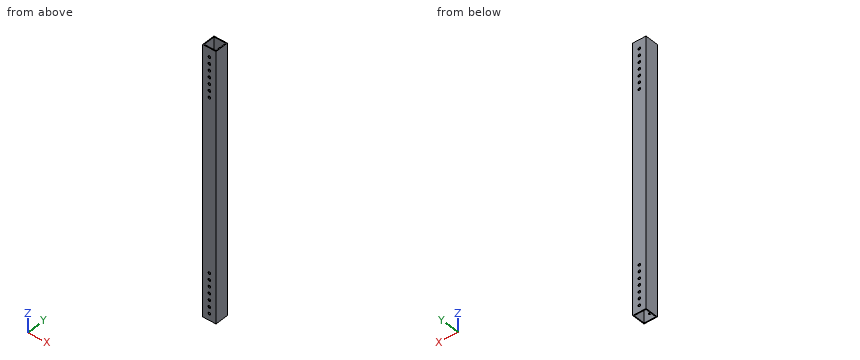
from build123d import *

# Parameters (mm, degrees)
SKETCH1_W               = 25.4
SKETCH1_H               = 25.4
BOSS_EXTRUDE1_DEPTH     = 256.145698528
SHELL1_T                = -1.5875
CUT_EXTRUDE1_DEPTH      = 257.774607145
CUT_EXTRUDE1_DEPTH_BACK = 257.774607145
SKETCH3_R               = 2.4892


with BuildPart() as part:
    # Sketch1 → Boss-Extrude1 (new, symmetric)
    with BuildSketch(Plane.XY):
        Rectangle(SKETCH1_W, SKETCH1_H)
    extrude(amount=BOSS_EXTRUDE1_DEPTH, both=True)

    # Shell1
    shell1_openings = [part.faces().sort_by_distance(p)[0] for p in [
        (0, 0, 256.145698528),
        (0, 0, -256.145698528),
    ]]
    offset(amount=SHELL1_T, openings=shell1_openings, kind=Kind.INTERSECTION)

    # Sketch3 → Cut-Extrude1 (cut, two sides: drawn at the far end of the back side and taken through both)
    with BuildSketch(Plane(origin=(0, 0, 0), x_dir=(1, 0, 0), z_dir=(0, 1, 0)).offset(-CUT_EXTRUDE1_DEPTH_BACK)):
        with Locations(Location((0, 243.445698528, 0), (0, 0, 270))):
            Circle(SKETCH3_R)
        with Locations(Location((0, 230.745698528, 0), (0, 0, 270))):
            Circle(SKETCH3_R)
        with Locations(Location((0, 218.045698528, 0), (0, 0, 270))):
            Circle(SKETCH3_R)
        with Locations(Location((0, 205.345698528, 0), (0, 0, 270))):
            Circle(SKETCH3_R)
        with Locations(Location((0, 192.645698528, 0), (0, 0, 270))):
            Circle(SKETCH3_R)
        with Locations(Location((0, 179.945698528, 0), (0, 0, 270))):
            Circle(SKETCH3_R)
        with Locations(Location((0, 167.245698528, 0), (0, 0, 270))):
            Circle(SKETCH3_R)
        with Locations(Location((0, -162.954301472, 0), (0, 0, 270))):
            Circle(SKETCH3_R)
        with Locations(Location((0, -175.654301472, 0), (0, 0, 270))):
            Circle(SKETCH3_R)
        with Locations(Location((0, -188.354301472, 0), (0, 0, 270))):
            Circle(SKETCH3_R)
        with Locations(Location((0, -201.054301472, 0), (0, 0, 270))):
            Circle(SKETCH3_R)
        with Locations(Location((0, -213.754301472, 0), (0, 0, 270))):
            Circle(SKETCH3_R)
        with Locations(Location((0, -226.454301472, 0), (0, 0, 270))):
            Circle(SKETCH3_R)
        with Locations(Location((0, -239.154301472, 0), (0, 0, 270))):
            Circle(SKETCH3_R)
    extrude(amount=CUT_EXTRUDE1_DEPTH + CUT_EXTRUDE1_DEPTH_BACK, mode=Mode.SUBTRACT)


solid = part.part
Geometry: final body of the model. Coordinates: model frame, mm. Round coordinates to 2 decimals unless told otherwise and drop trailing zeros. Order: outer loops, then holes, each group sorted by start corner. A loop starts at its lowest first (then second) coordinate and runs counter-clockwise, first axis right, second up.
Q1. Material intervals for probe 1 along X at (y, z) = (1, -166.5), sorted ascending.
Result sheet:
probe 1: x = -12.7 to -11.11, 11.11 to 12.7
Q2. Section A-A, the plane x = -6.75. Output: boundary loops of the cut face in (y, z).
Result sheet:
outline: (-12.7, -256.15) - (-11.11, -256.15) - (-11.11, 256.15) - (-12.7, 256.15) - close; (11.11, -256.15) - (12.7, -256.15) - (12.7, 256.15) - (11.11, 256.15) - close
Q3. Pin query (flat end, axial travel): pin 1 (8 mm diameter, centred on x = 0, z = -230.75, fed in from -Y). Return the tip coordinate at first contact, or that it passes through.
Result sheet:
pin 1: stops at y = -12.7
Q4. Section B-B, the plane z = 68. Output: boundary loops of the cut face in (x, y).
Result sheet:
outline: (-12.7, -12.7) - (12.7, -12.7) - (12.7, 12.7) - (-12.7, 12.7) - close; hole (-11.11, -11.11) - (11.11, -11.11) - (11.11, 11.11) - (-11.11, 11.11) - close
